from build123d import *

# Parameters (mm, degrees)
BOSS_EXTRUDE1_DEPTH      = 6.35
BOSS_EXTRUDE1_DEPTH_BACK = 6.35
SKETCH2_W                = 292.995908675
SKETCH2_H                = 3.175
CUT_EXTRUDE1_DEPTH       = 38.1
SKETCH3_W                = 146.05
SKETCH3_H                = 3.175
CUT_EXTRUDE2_DEPTH       = 38.1
CUT_EXTRUDE3_DEPTH       = 3.175
CUT_EXTRUDE4_DEPTH       = 3.175
CUT_EXTRUDE5_DEPTH       = 157.099
CUT_EXTRUDE6_DEPTH       = 339.217
CUT_EXTRUDE6_DEPTH_BACK  = 157.099
SKETCH9_W                = 50.8
SKETCH9_H                = 19.05
CUT_EXTRUDE7_DEPTH       = 21.59
SKETCH11_W               = 6
SKETCH11_H               = 19.05
SKETCH11_W_2             = 0.965000048
CUT_EXTRUDE10_DEPTH      = 366.729881683


with BuildPart() as part:
    # Sketch1 → Boss-Extrude1 (new, two sides: drawn at the far end of the back side and taken through both)
    with BuildSketch(Plane(origin=(0, 0, 0), x_dir=(1, 0, 0), z_dir=(0, 1, 0)).offset(-BOSS_EXTRUDE1_DEPTH_BACK)):
        Polygon((-406.4, 0), (0, 0), (0, 146.05), (-152.4, 146.05), align=None)
    extrude(amount=BOSS_EXTRUDE1_DEPTH + BOSS_EXTRUDE1_DEPTH_BACK)

    # Sketch2 → Cut-Extrude1 (cut)
    with BuildSketch(Plane(origin=(-100.979614843, 0, -175.616721465), x_dir=(-0.8669063030575352, 0, 0.49847112425808277), z_dir=(-0.4984711242580827, 0, -0.8669063030575351))):
        with Locations((205.812767226, 4.7625)):
            Rectangle(SKETCH2_W, SKETCH2_H)
        with Locations((205.812767226, -4.7625)):
            Rectangle(SKETCH2_W, SKETCH2_H)
    extrude(amount=-CUT_EXTRUDE1_DEPTH, mode=Mode.SUBTRACT)

    # Sketch3 → Cut-Extrude2 (cut)
    with BuildSketch(Plane(origin=(0, 0, 0), x_dir=(0, 0, -1), z_dir=(1, 0, 0))):
        with Locations((73.025, 4.7625)):
            Rectangle(SKETCH3_W, SKETCH3_H)
        with Locations((73.025, -4.7625)):
            Rectangle(SKETCH3_W, SKETCH3_H)
    extrude(amount=-CUT_EXTRUDE2_DEPTH, mode=Mode.SUBTRACT)

    # Sketch4 → Cut-Extrude3 (cut)
    with BuildSketch(Plane(origin=(0, 6.35, 0), x_dir=(1, 0, 0), z_dir=(0, 1, 0))):
        Polygon((-133.408250166, 113.020869854), (-75.966284694, 146.05), (-152.4, 146.05), align=None)
    extrude(amount=-CUT_EXTRUDE3_DEPTH, mode=Mode.SUBTRACT)

    # Sketch5 → Cut-Extrude4 (cut)
    with BuildSketch(Plane.XZ.offset(6.35)):
        Polygon((-133.408250166, -113.020869854), (-75.966284694, -146.05), (-152.4, -146.05), align=None)
    extrude(amount=-CUT_EXTRUDE4_DEPTH, mode=Mode.SUBTRACT)

    # Sketch6 → Cut-Extrude5 (cut)
    with BuildSketch(Plane(origin=(0, 0, -146.05), x_dir=(-1, 0, 0), z_dir=(0, 0, -1))):
        Polygon((38.1, -3.175), (43.18, -3.175), (43.18, -6.35), (38.1, -6.35), (0, -6.35), (0, 6.35), (38.1, 6.35), (43.18, 6.35), (43.18, 3.175), (38.1, 3.175), (38.1, 1.5875), (35.56, 1.5875), (35.56, -1.5875), (38.1, -1.5875), align=None)
    extrude(amount=-CUT_EXTRUDE5_DEPTH, mode=Mode.SUBTRACT)

    # Sketch8 → Cut-Extrude6 (cut, two sides: drawn at the far end of the back side and taken through both)
    with BuildSketch(Plane(origin=(-51.420385157, 0, 29.566721465), x_dir=(0.49847112425808243, 0, 0.8669063030575355), z_dir=(-0.8669063030575355, 0, 0.49847112425808243)).offset(-CUT_EXTRUDE6_DEPTH_BACK)):
        Polygon((-164.478664898, 3.175), (-159.398664898, 3.175), (-159.398664898, 6.35), (-164.478664898, 6.35), (-202.578664898, 6.35), (-202.578664898, -6.35), (-164.478664898, -6.35), (-159.398664898, -6.35), (-159.398664898, -3.175), (-164.478664898, -3.175), (-164.478664898, -1.5875), (-167.018664898, -1.5875), (-167.018664898, 1.5875), (-164.478664898, 1.5875), align=None)
    extrude(amount=CUT_EXTRUDE6_DEPTH + CUT_EXTRUDE6_DEPTH_BACK, mode=Mode.SUBTRACT)

    # Sketch9 → Cut-Extrude7 (cut)
    with BuildSketch(Plane(origin=(0, 6.35, 0), x_dir=(1, 0, 0), z_dir=(0, 1, 0))):
        with Locations((-25.4, 136.525)):
            Rectangle(SKETCH9_W, SKETCH9_H)
    extrude(amount=-CUT_EXTRUDE7_DEPTH, mode=Mode.SUBTRACT)

    # Sketch11 → Cut-Extrude10 (cut, through all)
    with BuildSketch(Plane(origin=(0, 6.35, 0), x_dir=(1, 0, 0), z_dir=(0, 1, 0))):
        with Locations((-54.765000048, 136.525)):
            Rectangle(SKETCH11_W, SKETCH11_H)
        with Locations((-51.282500024, 136.525)):
            Rectangle(SKETCH11_W_2, SKETCH11_H)
    extrude(amount=-CUT_EXTRUDE10_DEPTH, mode=Mode.SUBTRACT)


solid = part.part
Can you work these out from the model? Positions are in its coordinate system, mm. A direction names the side the tool comes from. Coordinates: 2 decimals unless noted, no trailing zeros. Return JSON: item names as keys, results as strings. Group by question number.
Item 1: I'm going to push flat-ended pins straight in: pin 1 Ø1.3 at (x, z) = (-37, -36) entering from -Y; pin 2 Ø0.8 at (y, z) = (2.5, -59.5) entering from +X; pin 3 Ø5 at (y, z) = (1, -80.5) entering from -X. Where does each tip first touch, or does it pass through?
Item 2: Please list where these lines run through material, in increasing order: probe 1 along Z at (x, y) = (-183, -3); probe 2 along Z at (x, y) = (-310, 3.75); probe 3 along Y at (x, z) = (-156, -102.5).
Item 3: Which directions (+Z, -Z, +X, -X, +Y, -Y) give clear straight access to the entire face, cutting with the end or side of a thin tool? Please do faces 1 (the face through (-204, 1.588, -74)), 2 (the face through (-196, -3.175, -74)), 3 (the face through (-41, 3.175, -64)), 4 (the face through (-41, -3.175, -64)), 5 (the face through (-57.765, 0, -136)).
Return value:
{
 "1": {"pin 1": "stops at y = -1.59", "pin 2": "stops at x = -38.1", "pin 3": "stops at x = -199.41"},
 "2": {"probe 1": "z = -84.51 to 0", "probe 2": "z = -5.62 to 0", "probe 3": "y = -1.59 to 1.59"},
 "3": {"face 1": "-Z, -X, +Y", "face 2": "-Z, -X, -Y", "face 3": "+Z, -Z, +X, +Y", "face 4": "+Z, -Z, +X, -Y", "face 5": "-Z, +X, +Y, -Y"}
}
